Can you work these out from the model? Positions are in its coordinate system, mm. A direction names the side the tool comes from. Give positions to 0.01 mm unless a question says otherwise; leave off trailing zeros. Order: outer loops, then holes, each group sorted by start corner. A loop starts at its lowest first (then second) coordinate and runs counter-clockwise, first axis right, second up. Notation, with made-up numbers: (36, 39) - (45, 39) arc R27 cw to (45, 78) - close; hole circle Ø7 at (8, 17.5). An arc over 180 degrees is marked (long way). Answer as a JSON object with one key per item and string values.
```python
from build123d import *

# Parameters (mm, degrees)
SKETCH1_W           = 250
SKETCH1_H           = 25
BOSS_EXTRUDE1_DEPTH = 50
SKETCH2_W           = 220
SKETCH2_H           = 10
CUT_EXTRUDE1_DEPTH  = 35
SKETCH3_R           = 25
BOSS_EXTRUDE2_DEPTH = 49
LPATTERN1_COUNT     = 3
LPATTERN1_PITCH     = 100.5
SKETCH7_R           = 12.5
CUT_EXTRUDE2_DEPTH  = 250
SKETCH8_W           = 250
SKETCH8_H           = 19.943004224
CUT_EXTRUDE3_DEPTH  = 5
SKETCH10_R          = 26.5
CUT_EXTRUDE4_DEPTH  = 52
SKETCH15_R          = 26.5
CUT_EXTRUDE5_DEPTH  = 52


with BuildPart() as part:
    # Sketch1 → Boss-Extrude1 (new body)
    with BuildSketch(Plane.XY):
        with Locations((110, 12.5)):
            Rectangle(SKETCH1_W, SKETCH1_H)
    extrude(amount=BOSS_EXTRUDE1_DEPTH)

    # Sketch2 → Cut-Extrude1 (cut)
    with BuildSketch(Plane(origin=(0, 0, 0), x_dir=(-1, 0, 0), z_dir=(0, 0, -1))):
        with Locations((-110, 5)):
            Rectangle(SKETCH2_W, SKETCH2_H)
    extrude(amount=-CUT_EXTRUDE1_DEPTH, mode=Mode.SUBTRACT)

    # Sketch3 → Boss-Extrude2 (add)
    with BuildSketch(Plane.ZY.offset(15)):
        with Locations((40.462008594, 39.281822702)):
            Circle(SKETCH3_R)
    boss_extrude2 = extrude(amount=-BOSS_EXTRUDE2_DEPTH)

    # LPattern1: Boss-Extrude2 ×3
    with Locations(*[(i * LPATTERN1_PITCH, 0, 0) for i in range(1, LPATTERN1_COUNT)]):
        add(boss_extrude2)

    # Sketch7 → Cut-Extrude2 (cut)
    with BuildSketch(Plane.ZY.offset(15)):
        with Locations((40.272500431, 39.79236851)):
            Circle(SKETCH7_R)
    extrude(amount=-CUT_EXTRUDE2_DEPTH, mode=Mode.SUBTRACT)

    # Sketch8 → Cut-Extrude3 (cut)
    with BuildSketch(Plane(origin=(0, 25, 0), x_dir=(1, 0, 0), z_dir=(0, 1, 0))):
        with Locations((110, -9.971502112)):
            Rectangle(SKETCH8_W, SKETCH8_H)
    extrude(amount=-CUT_EXTRUDE3_DEPTH, mode=Mode.SUBTRACT)

    # Sketch10 → Cut-Extrude4 (cut)
    with BuildSketch(Plane.ZY.offset(-85.5)):
        with Locations((40.272500431, 39.79236851)):
            Circle(SKETCH10_R)
    extrude(amount=CUT_EXTRUDE4_DEPTH, mode=Mode.SUBTRACT)

    # Sketch15 → Cut-Extrude5 (cut)
    with BuildSketch(Plane.ZY.offset(-186)):
        with Locations((40.272500431, 39.79236851)):
            Circle(SKETCH15_R)
    extrude(amount=CUT_EXTRUDE5_DEPTH, mode=Mode.SUBTRACT)


solid = part.part
```
Q1. If we section it at D-D, the plane z = 4: Please give me the cut outline in (x, y), then the cut area to 3 significant figures.
Recorded:
{"outline": "(-15, 0) - (0, 0) - (0, 10) - (220, 10) - (220, 0) - (235, 0) - (235, 20) - (-15, 20) - close", "area": "2,800 mm^2"}
Q2. I'm going to push flat-ended pins straight in: pin 1 Ø12 at (x, y) = (33, 9.5) entering from +Z; pin 2 Ø10 at (x, z) = (63, 11.5) entering from +Y; pin 3 Ø3 at (x, y) = (75, 7) entering from -Z. Where does each tip first touch, or does it pass through?
Recorded:
{"pin 1": "stops at z = 50", "pin 2": "stops at y = 20", "pin 3": "stops at z = 35"}
Q3. Which directions (+Z, -Z, +X, -X, +Y, -Y) give clear straight access to the entire face, cutting with the end or side of a thin tool? Please do faces 1 (the face through (108, 8, 50)), 2 (the face through (108, 20, 10)), 3 (the face through (220, 5, 17)).
Recorded:
{"face 1": "+Z, +X, -X, -Y", "face 2": "-Z, +X, -X", "face 3": "-Z, -Y"}
Q4. If we section it at C-C, the plane y = 45: Please give me the cut outline in (x, z), then the cut area to 3 significant figures.
Recorded:
{"outline": "(-15, 16.12) - (33.5, 16.12) - (33.5, 28.91) - (-15, 28.91) - close; (-15, 51.64) - (33.5, 51.64) - (33.5, 64.8) - (-15, 64.8) - close; (85.5, 16.12) - (134, 16.12) - (134, 28.91) - (85.5, 28.91) - close; (85.5, 51.64) - (134, 51.64) - (134, 64.8) - (85.5, 64.8) - close; (186, 16.12) - (235, 16.12) - (235, 28.91) - (186, 28.91) - close; (186, 51.64) - (235, 51.64) - (235, 64.8) - (186, 64.8) - close", "area": "3,790 mm^2"}
Q5. I need wall thicknesses on L1, parallel to X at y = 45.5, z = 59; L2, parallel to Y at x = -2, z = 40; L3, parallel to Z at x = 132.5, y = 5. Which ranges of each line are inside material? Lowest first, please.
Recorded:
{"L1": "x = -15 to 33.5, 85.5 to 134, 186 to 235", "L2": "y = 0 to 27.3, 52.29 to 64.28", "L3": "z = 35 to 50"}
Q6. If we section it at B-B, the plane z = 58: Please give me the cut outline in (x, y).
Recorded:
{"outline": "(-15, 21.47) - (33.5, 21.47) - (33.5, 57.1) - (-15, 57.1) - close; (85.5, 21.47) - (134, 21.47) - (134, 57.1) - (85.5, 57.1) - close; (186, 21.47) - (235, 21.47) - (235, 57.1) - (186, 57.1) - close"}
Q7. We'd pull the mould along Y, two halves only. Please class faces 4 (the face through (210.16, 27.59, 37.56)), 5 (the face through (59.86, 14.17, 33.51)), 6 (the face through (-15, 25, 32)): released by +Y, released by -Y, zero draft, split by the parting line, or undercut.
Recorded:
{"face 4": "undercut", "face 5": "released by +Y", "face 6": "zero draft"}
Q8. If we section it at A-A, the plane y = 59.5: Please give me the cut outline in (x, z), then the cut area to 3 significant figures.
Recorded:
{"outline": "(-15, 25.76) - (33.5, 25.76) - (33.5, 55.17) - (-15, 55.17) - close; (85.5, 25.76) - (134, 25.76) - (134, 55.17) - (85.5, 55.17) - close; (186, 25.76) - (235, 25.76) - (235, 55.17) - (186, 55.17) - close", "area": "4,290 mm^2"}
